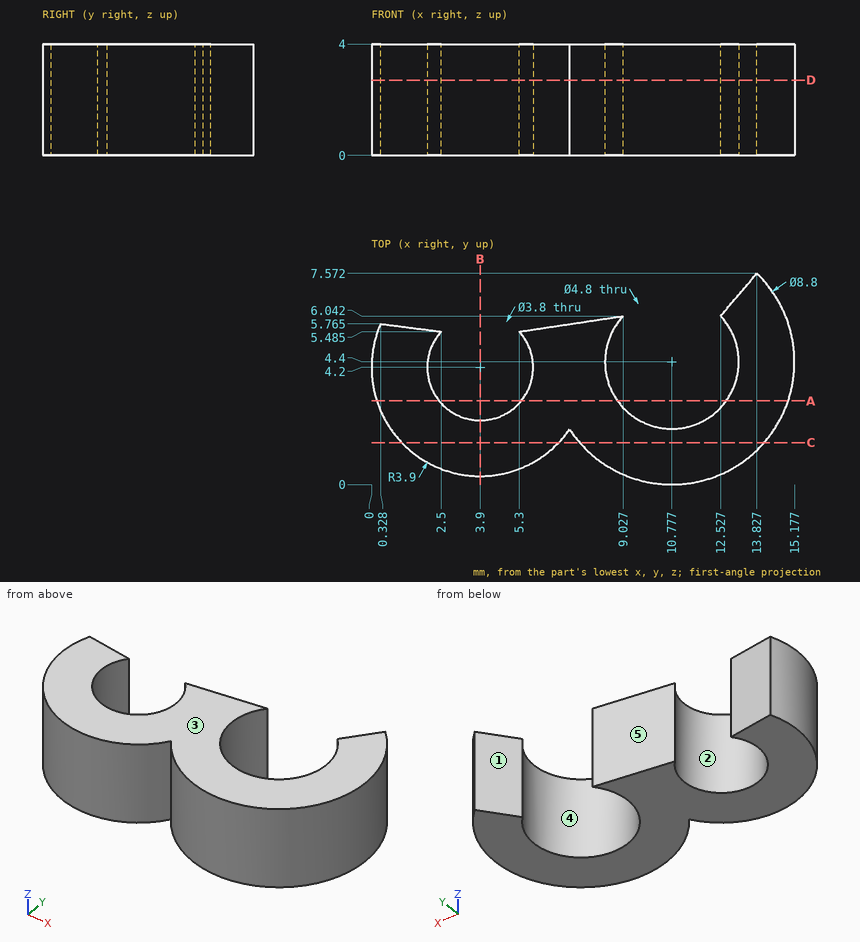
Geometry: see drawing. Coordinates: mm, zero at the bounding-box minimum. A direction names the side the tool comes from. Coordinates: 2 decimals unless noted, no trailing zeros. Loops run counter-clockwise (first coordinate to the right, second up) from the corner with the lowest first, then second, coordinate; pieces in that order, holes last. Notation, with made-up numbers: M -11.75,-18 L 14.25,-18 A15 cw 14.25,-11 Z; hole C 41,35.5 d9. An arc over 180 degrees is marked long. Put each result on its own line as item: value. Start each with the question number.
1) Pull-direction query (Y, two-part tool) for the marked faces 1, 2 and 3; classes: pulls with the +Y half, pulls with the -Y half, needs draft (parallel to the pull), parting line crosses it, or undercut.
2) Cut plane D-D on z = 2.7. Return the cut outline in (x, y) (1 decimal).
3) Ray query, L1, parallel to X at y = 5.25, z = 2.7 (1 decimal); L2, parallel to X at y = 4.75, z = 2.05; L3, parallel to X at y = 1, z = 0.95 (1 decimal). Return the intervals inside material, ascending. Write a range as from..to.
4) Reachability of the marked faces 4 and 5 from +Z, -Z, +X, -X, +Y, -Y: full face, straight path, thin tool, end or side. Return the list, or none.
5) Cut plane C-C on y = 1.5. Return the cut outline in (x, z) (1 decimal).
6) Cut plane A-A on y = 3. Return the cut outline in (x, z).
7) Cut plane B-B on x = 3.9. Return the cut outline in (y, z).
The answers:
1. face 1: pulls with the +Y half
1. face 2: undercut
1. face 3: needs draft
2. outline: M 0.3,5.8 A3.9 ccw 7.1,2 A4.4 ccw long 13.8,7.6 L 12.5,6 A2.4 cw long 9,6 L 5.3,5.5 A1.9 cw long 2.5,5.5 Z
3. L1: x = 0.1..2.3, 5.5..8.5, 13..15.1
3. L2: x = 0.04..2.08, 5.72..8.4, 13.15..15.16
3. L3: x = 1.7..6.1, 8..13.6
4. face 4: +Z, -Z
4. face 5: +Z, -Z, +Y
5. outline: M 1.1,0 L 6.7,0 L 6.7,4 L 1.1,4 Z; M 7.5,0 L 14.1,0 L 14.1,4 L 7.5,4 Z
6. outline: M 0.19,0 L 2.43,0 L 2.43,4 L 0.19,4 Z; M 5.37,0 L 8.83,0 L 8.83,4 L 5.37,4 Z; M 12.73,0 L 14.95,0 L 14.95,4 L 12.73,4 Z
7. outline: M 0.3,0 L 2.3,0 L 2.3,4 L 0.3,4 Z
